Could you check a few things on this drawing? It's one solid part, dimensions in mm from its lowest x, y, z. A direction names the side the tool comes from. Coordinates: 2 decimals unless noted, no trailing zeros. Order: outer loops, then holes, each group sorted by start corner. A loop starts at its lowest first (then second) coordinate and runs counter-clockwise, first axis right, second up.
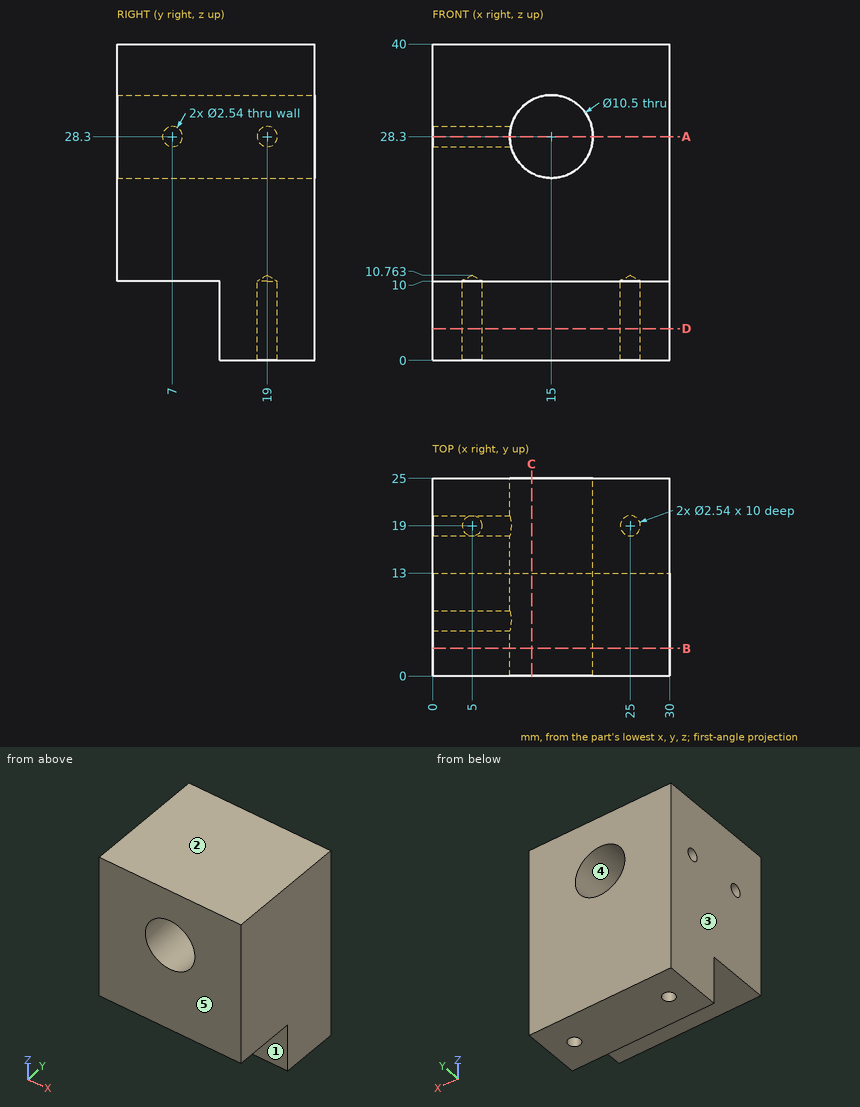
Q1. If we section it at D-D on z = 4: Write out the boundary of the cut face in (x, y), then the cut area to 3 significant figures.
Q2. Will these pins go through, and if not, where does the flat tip stop? pin 1 (4 mm diameter, centred on x = 6, y = 3.5, fed in from -Z); pin 2 (5 mm diameter, centred on x = 18.5, z = 7, fed in from -Y).
Q3. I need wall thicknesses on L1, parallel to Y at x = 5, z = 5.75; L2, parallel to Y at x = 2.25, z = 28.3; L3, parallel to Z at x = 27, y = 12.25. Which ranges of each line are inside material? Lowest first, please.
Q4. If we section it at B-B on y = 3.5: Write out the boundary of the cut face in (x, z), then the cut area to 3 significant figures.
Q5. For the marked faces 1 and 2, which set-ups out of +Z, -Z, +X, -X, +Y, -Y let a thin tool reach every point of the face, with its end or its side?
Q6. We'd pull the mould along X, two halves only. Please class the marked faces 3, 4 and 5: pulls with the +X half, pulls with the -X half, needs draft (parallel to the pull), parting line crosses it, or undercut.
Q7. If we section it at C-C on x = 12.5: Write out the boundary of the cut face in (y, z), then the cut area to 3 significant figures.
Q8. If we section it at A-A on z = 28.3: Write out the boundary of the cut face in (x, y), then the cut area to 3 significant figures.
Reply:
1. outline: (0, 13) - (30, 13) - (30, 25) - (0, 25) - close; hole circle Ø2.54 at (5, 19); hole circle Ø2.54 at (25, 19)
1. area: 350 mm2
2. pin 1: stops at z = 10
2. pin 2: stops at y = 13
3. L1: y = 13 to 17.73, 20.27 to 25
3. L2: y = 0 to 5.73, 8.27 to 17.73, 20.27 to 25
3. L3: z = 10 to 40
4. outline: (0, 10) - (30, 10) - (30, 40) - (0, 40) - close; hole circle Ø10.5 at (15, 28.3)
4. area: 813 mm2
5. face 1: -Z, +X, -X, -Y
5. face 2: +Z, +X, -X, +Y, -Y
6. face 3: pulls with the -X half
6. face 4: undercut
6. face 5: needs draft
7. outline: (0, 10) - (13, 10) - (13, 0) - (25, 0) - (25, 23.68) - (0, 23.68) - close; (0, 32.92) - (25, 32.92) - (25, 40) - (0, 40) - close
7. area: 639 mm2
8. outline: (0, 0) - (9.75, 0) - (9.75, 5.73) - (0, 5.73) - close; (0, 8.27) - (9.75, 8.27) - (9.75, 17.73) - (0, 17.73) - close; (0, 20.27) - (9.75, 20.27) - (9.75, 25) - (0, 25) - close; (20.25, 0) - (30, 0) - (30, 25) - (20.25, 25) - close
8. area: 438 mm2
